Verification items for this drawing (mm, ordinates from the low corner). A direction names the side the tool comes from. Give positions to 0.01 mm unless a question says otherwise; leave off trailing zeros. Order: outer loops, then holes, each group sorted by start corner. A loop starts at its lowest first (then second) coordinate and runs counter-clockwise, first axis right, second up. Notation, with made-up numbers: M 34.5,59.25 L 90.5,59.25 A8 ccw 90.5,67.25 Z; hole C 84,19 d8. An arc over 180 degrees is marked long. Answer as a JSON object with one key per item and string values.
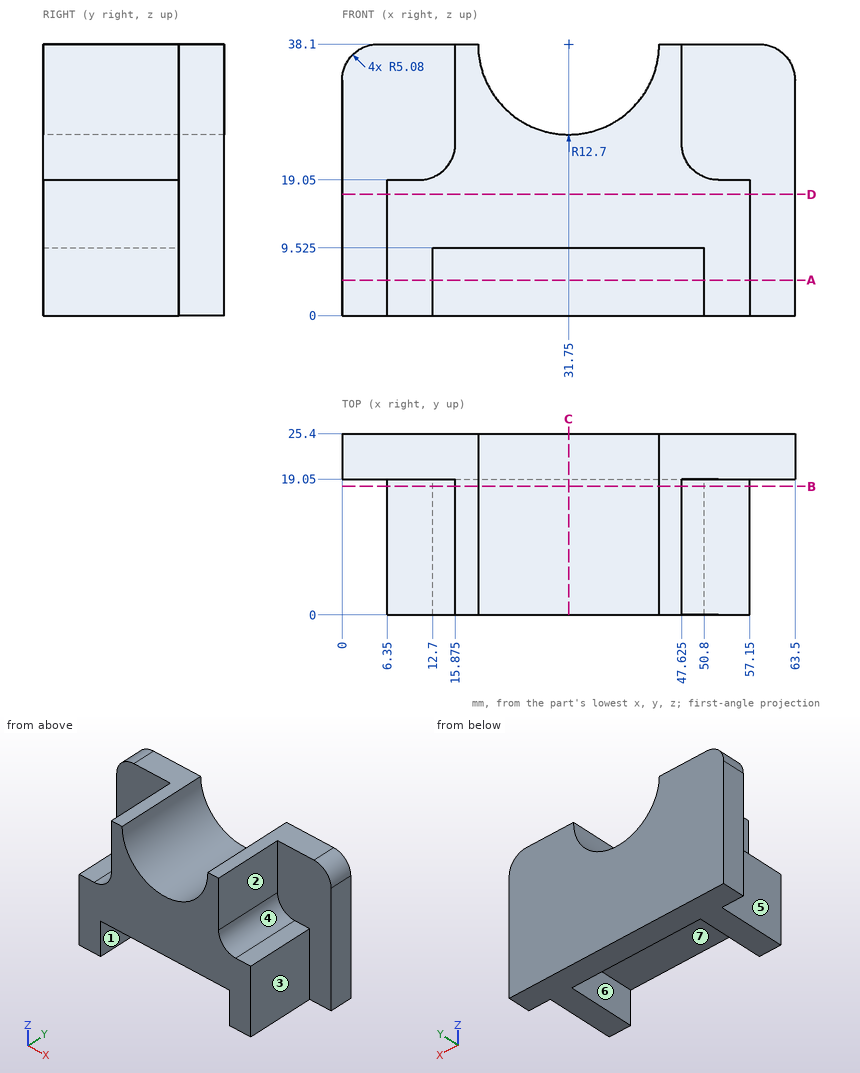
Q1. Release check for a two-part mould opening along X. For the marked faces 4, 5, 6 and 7 record: +X half, -X half, draft (parallel to the pull), parting line (faces both ways), or undercut.
Resolved:
{"face 4": "+X half", "face 5": "-X half", "face 6": "undercut", "face 7": "undercut"}
Q2. Section check C-C on x = 31.75. Record the cut outline in (y, z) (3 decimals).
Resolved:
{"outline": "M 0,9.525 L 19.05,9.525 L 19.05,0 L 25.4,0 L 25.4,25.4 L 0,25.4 Z"}
Q3. Section check D-D on z = 17. Record the cut outline in (x, y).
Resolved:
{"outline": "M 0,19.05 L 6.35,19.05 L 6.35,0 L 57.15,0 L 57.15,19.05 L 63.5,19.05 L 63.5,25.4 L 0,25.4 Z"}
Q4. Material ranges on L1, parallel to X at y = 6, z = 2; L2, parallel to Y at x = 3.5, z = 3; L3, parallel to X at y = 7.25, z = 14.5, recorded low to high.
Resolved:
{"L1": "x = 6.35 to 12.7, 50.8 to 57.15", "L2": "y = 19.05 to 25.4", "L3": "x = 6.35 to 57.15"}
Q5. Gauge pin test, flat ends, axial feed: pin 1 Ø8 at (x, y) = (16.5, 17) entering from -Z; pin 2 Ø12 at (x, y) = (35, 3) entering from -Z (3 decimals); pin 3 Ø5 at (x, z) = (7.5, 26.5) entering from -Y; pin 4 Ø5 at (y, z) = (15.5, 31.5) entering from +X (3 decimals). Record the tip position at first contact, or that the pin passes through.
Resolved:
{"pin 1": "stops at z = 0", "pin 2": "stops at z = 9.525", "pin 3": "stops at y = 19.05", "pin 4": "stops at x = 47.625"}
Q6. Section check B-B on y = 18. Record the cut outline in (x, z) (3 decimals), then the cut area to 3 significant figures.
Resolved:
{"outline": "M 6.35,0 L 12.7,0 L 12.7,9.525 L 50.8,9.525 L 50.8,0 L 57.15,0 L 57.15,19.05 L 52.705,19.05 A5.08 cw 47.625,24.13 L 47.625,38.1 L 44.45,38.1 A12.7 cw 19.05,38.1 L 15.875,38.1 L 15.875,24.13 A5.08 cw 10.795,19.05 L 6.35,19.05 Z", "area": "967 mm²"}
Q7. Tool access check on the marked faces 1, 2 and 3. Record the directions out of +Z, -Z, +X, -X, +Y, -Y that give a thin tool (end or side, any length) a straight path to the whole face; none if there is none.
Resolved:
{"face 1": "-Z, -Y", "face 2": "+Z, +X, -Y", "face 3": "+Z, -Z, +X, -Y"}
Q8. Section check A-A on z = 5. Record the cut outline in (x, y).
Resolved:
{"outline": "M 0,19.05 L 6.35,19.05 L 6.35,0 L 12.7,0 L 12.7,19.05 L 50.8,19.05 L 50.8,0 L 57.15,0 L 57.15,19.05 L 63.5,19.05 L 63.5,25.4 L 0,25.4 Z"}
